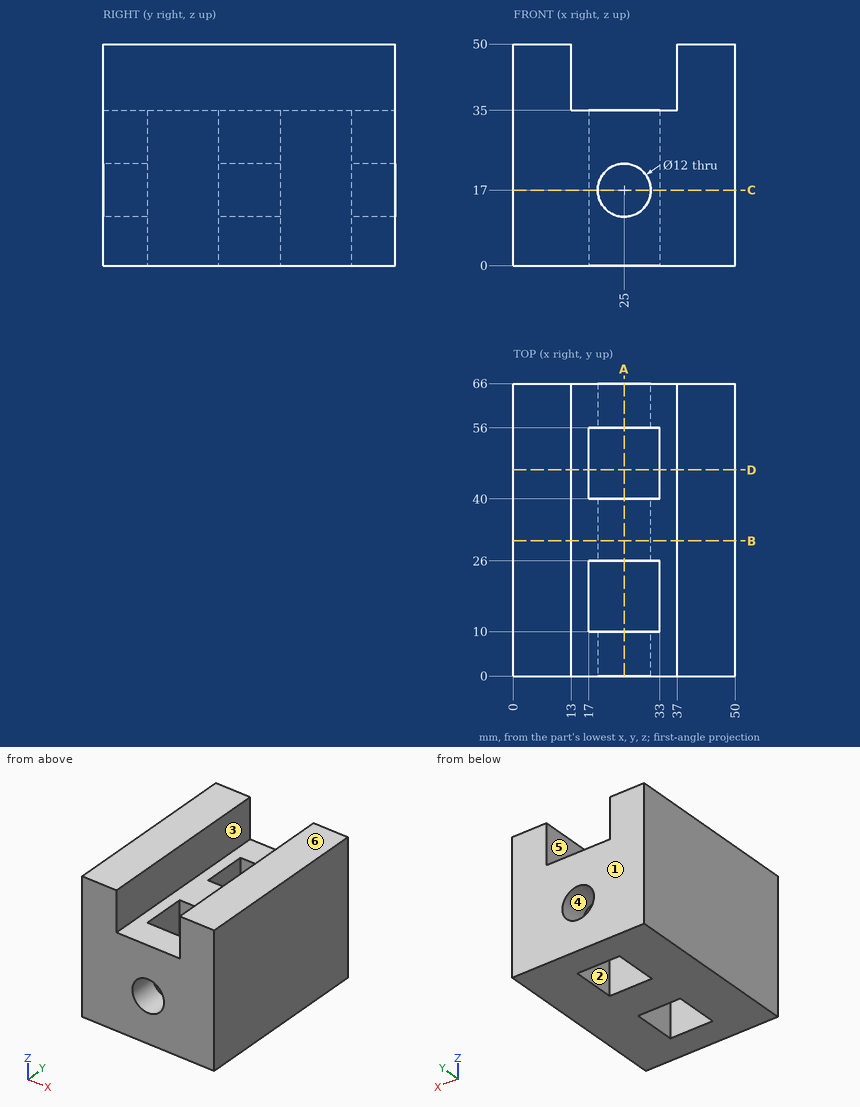
Input: dimensioned drawing with shaded views. Units: mm. Origin: part minimum x, y, z. A direction names the side the tool comes from. Coordinates: 2 decimals unless noted, no trailing zeros. Order: outer loops, then holes, each group sorted by start corner. A loop starts at its lowest first (then second) coordinate and runs counter-clockwise, first axis right, second up. Notation, with made-up numbers: M 46,22 L 91,22 A22 cw 91,51 Z; hole C 87.25,18.5 d2. An arc over 180 degrees is marked long. Write each question's results on one line, items separated by ' | '. Start each with the question number.
Item 1: Set-up query: the marked faces 1, 2 and 3. Return all of +Z, -Z, +X, -X, +Y, -Y with unobstructed straight access to the full face (end or side cutting, diameter ignored); none if empty.
Item 2: Cut plane D-D (y = 46.5). Return loops of the section in (x, z), and give its area (3 significant figures).
Item 3: Cut plane B-B (y = 30.5). Return loops of the section in (x, z).
Item 4: Cut plane A-A (x = 25). Return loops of the section in (y, z).
Item 5: Cut plane C-C (z = 17). Return loops of the section in (x, y).
Item 6: Draft query along Z for the marked faces 4, 5 and 6. Return one class per face: pulls with the +Z half, pulls with the -Z half, needs draft (parallel to the pull), parting line crosses it, or undercut.
Item 7: Line query: probe 1 along Y at (x, z) = (25, 5); probe 2 along X at (y, z) = (5.5, 17); probe 3 along Z at (x, y) = (25, 63). Output: solid intervals per line, ascending.
Item 8: First-contact query: pin 1 Ø8 at (y, z) = (46, 9.5) entering from -X; pin 2 Ø12 at (x, y) = (21, 47.5) entering from +Z. Flat tips, straight axial feed; report the tip coordinate or a pass-through.
Checked values:
1) face 1: +Z, -Z, +X, -X, +Y | face 2: +Z, -Z | face 3: +Z, +Y, -Y
2) outline: M 0,0 L 17,0 L 17,35 L 13,35 L 13,50 L 0,50 Z; M 33,0 L 50,0 L 50,50 L 37,50 L 37,35 L 33,35 Z | area: 1,580 mm2
3) outline: M 0,0 L 50,0 L 50,50 L 37,50 L 37,35 L 13,35 L 13,50 L 0,50 Z; hole C 25,17 d12
4) outline: M 0,0 L 10,0 L 10,11 L 0,11 Z; M 0,23 L 10,23 L 10,35 L 0,35 Z; M 26,0 L 40,0 L 40,11 L 26,11 Z; M 26,23 L 40,23 L 40,35 L 26,35 Z; M 56,0 L 66,0 L 66,11 L 56,11 Z; M 56,23 L 66,23 L 66,35 L 56,35 Z
5) outline: M 0,0 L 19,0 L 19,10 L 17,10 L 17,26 L 19,26 L 19,40 L 17,40 L 17,56 L 19,56 L 19,66 L 0,66 Z; M 31,0 L 50,0 L 50,66 L 31,66 L 31,56 L 33,56 L 33,40 L 31,40 L 31,26 L 33,26 L 33,10 L 31,10 Z
6) face 4: undercut | face 5: needs draft | face 6: pulls with the +Z half
7) probe 1: y = 0 to 10, 26 to 40, 56 to 66 | probe 2: x = 0 to 19, 31 to 50 | probe 3: z = 0 to 11, 23 to 35
8) pin 1: stops at x = 0 | pin 2: stops at z = 35
